from build123d import *

# Parameters (mm, degrees)
F0_W     = 70
F0_H     = 7
F1_DEPTH = 7
F2_R     = 2.5
F3_DEPTH = 5
F4_R     = 2.5
F5_DEPTH = 4


with BuildPart() as f1:
    # F0 (on Top) → F1 (new body)
    with BuildSketch(Plane.XY):
        with Locations((35, 3.5)):
            Rectangle(F0_W, F0_H)
    extrude(amount=F1_DEPTH)

    # F2 (on face) → F3 (cut)
    with BuildSketch(Plane.YZ.offset(70)):
        with Locations((3.5, 3.5)):
            Circle(F2_R)
    extrude(amount=-F3_DEPTH, mode=Mode.SUBTRACT)

    # F4 (on face) → F5 (join)
    with BuildSketch(Plane(origin=(0, 0, 0), x_dir=(0, -1, 0), z_dir=(-1, 0, 0))):
        with Locations((-3.5, 3.5)):
            Circle(F4_R)
    extrude(amount=F5_DEPTH)


solid = f1.part
Design review of the part built by this model. Coordinates are the model's own, in mm. A direction names the side the tool comes from. Coordinates: 2 decimals unless noted, no trailing zeros. Order: outer loops, then holes, each group sorted by start corner. A loop starts at its lowest first (then second) coordinate and runs counter-clockwise, first axis right, second up.
Item 1: The part is to be moulded in two halves that separate along Y. For faces 4 (the flat face through (-4, 4, 4)), 5 (the flat face through (35, 7, 3)), 6 (the cylindrical face through (67.535, 5.885, 4.251)), say which applies: pulls with the +Y half, pulls with the -Y half, needs draft (parallel to the pull), parting line crosses it, or undercut.
Item 2: For faces 1 (the cylindrical face through (-1.972, 1.115, 4.251)), 2 (the flat face through (70, 2, 1)), 3 (the flat face through (65, 3, 4)), list the 3-axis set-ups (+Z, -Z, +X, -X, +Y, -Y) from which the entire face can be reached by the end or side of a thin tool; tool diameter is ignored.
Item 3: For line 1 (Z direction, x = 67.2, y = 3.5); line 2 (X direction, y = 2, z = 0.5); line 3 (X direction, y = 2.25, z = 5.5), list the stretches that pass through material, from the lowest coordinate up.
Item 4: Take a section at A-A, the plane z = 3.5. Write out the cut boundary in (x, y), then the cut area to 3 significant figures.
The answers:
1. face 4: needs draft
1. face 5: pulls with the +Y half
1. face 6: undercut
2. face 1: -X
2. face 2: +Z, -Z, +X, +Y, -Y
2. face 3: +X
3. line 1: z = 0 to 1, 6 to 7
3. line 2: x = 0 to 70
3. line 3: x = -4 to 65
4. outline: (-4, 1) - (0, 1) - (0, 0) - (70, 0) - (70, 1) - (65, 1) - (65, 6) - (70, 6) - (70, 7) - (0, 7) - (0, 6) - (-4, 6) - close
4. area: 485 mm2
